Autodesk Inventor part; units mm, degrees
ref_plane "YZ Plane" through (0, 0, 0) normal (1, 0, 0) x (0, 1, 0)
ref_plane "XZ Plane" through (0, 0, 0) normal (0, 1, 0) x (-1, 0, 0)
ref_plane "XY Plane" through (0, 0, 0) normal (0, 0, 1) x (1, 0, 0)
sketch "草圖1" plane through (0, 0, 0) normal (0, 1, 0) x (-1, 0, 0)
  line L0 (4.2, 0) -> (4.2, -6)
  line L1 (4.2, -6) -> (0, -6)
  line L2 (0, -6) -> (1.2, -6)
  line L3 (1.2, -6) -> (1.2, -12)
  line L4 (1.2, -12) -> (0, -12)
  line L5 (-4.2, 0) -> (-4.2, -6)
  line L6 (-4.2, -6) -> (0, -6)
  line L7 (0, -6) -> (-1.2, -6)
  line L8 (-1.2, -6) -> (-1.2, -12)
  line L9 (-1.2, -12) -> (0, -12)
  line L10 (4.2, 0) -> (4.2, 6)
  line L11 (4.2, 6) -> (0, 6)
  line L12 (0, 6) -> (1.2, 6)
  line L13 (1.2, 6) -> (1.2, 12)
  line L14 (1.2, 12) -> (0, 12)
  line L15 (-4.2, 0) -> (-4.2, 6)
  line L16 (-4.2, 6) -> (0, 6)
  line L17 (0, 6) -> (-1.2, 6)
  line L18 (-1.2, 6) -> (-1.2, 12)
  line L19 (-1.2, 12) -> (0, 12)
  circle A0 centre (0, 0) radius 1.5
  dimension "d0" = 6
  dimension "d1" = 1.2
  dimension "d2" = 3
  dimension "d3" = 6
  dimension "d4" = 3
extrude "擠出1" add sketch "草圖1" along normal mid plane 3
properties part number "小零件1"
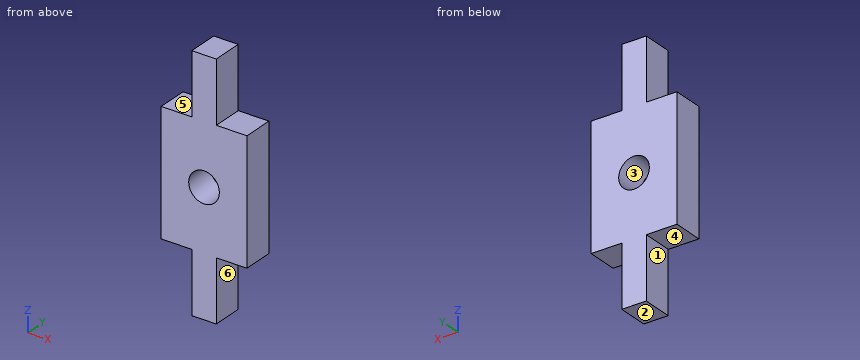
Source: CAD feature listing. Evaluate the final solid. Frame: model axes, mm. Face numbers are marked on the shaded views. A direction names the side the tool comes from. Give positions to 0.01 mm unless a question says otherwise; leave off trailing zeros. Write each loop counter-clockwise with the first axis right and the second up, starting at its lowest first coordinate (ties: lowest second). Pieces come first, ordered by that corner, then holes.
1. Material intervals for line 1 along Z through (x, y) = (0, 0.7); line 2 along Z through (x, y) = (2.75, -0.35); line 3 along X through (y, z) = (0.7, 1), sorted ascending.
2. First-contact query: pin 1 (1.5 mm diameter, centred on y = -0.5, z = 10.5, fed in from +X); pin 2 (0.9 mm diameter, centred on x = 3.5, y = 0.5, fed in from -Z); pin 3 (1.5 mm diameter, centred on y = 0.5, z = -9.5, fed in from -X). Flat tips, straight axial feed; report the tip coordinate or a pass-through.
3. Pull-direction query (X, two-part tool) for the marked faces 1, 2 and 3; classes: +X half, -X half, draft (parallel to the pull), parting line (faces both ways), or undercut.
4. Section query B-B (y = 0.15). Return the cut outline in (x, z).
5. Section query A-A (z = 0). Return the cut outline in (x, y), then the cut area to 3 significant figures.
6. Access query for the marked faces 4, 5 and 6. Directions: +Z, -Z, +X, -X, +Y, -Y. A direction counts if a zero-diameter tool reaches every point of the face in a straight line with its end or side. Return the directions, or none.
7. Section query D-D (x = -2). Return the cut outline in (y, z).
8. Section query C-C (x = 0). Return the cut outline in (y, z), then the cut area to 3 significant figures.
Output values:
1. line 1: z = -12 to -1.5, 1.5 to 12
1. line 2: z = -6 to 6
1. line 3: x = -4.2 to -1.12, 1.12 to 4.2
2. pin 1: stops at x = 1.2
2. pin 2: stops at z = -6
2. pin 3: stops at x = -1.2
3. face 1: -X half
3. face 2: draft
3. face 3: undercut
4. outline: (-4.2, -6) - (-1.2, -6) - (-1.2, -12) - (1.2, -12) - (1.2, -6) - (4.2, -6) - (4.2, 6) - (1.2, 6) - (1.2, 12) - (-1.2, 12) - (-1.2, 6) - (-4.2, 6) - close; hole circle Ø3 at (0, 0)
5. outline: (-4.2, -1.5) - (-1.5, -1.5) - (-1.5, 1.5) - (-4.2, 1.5) - close; (1.5, -1.5) - (4.2, -1.5) - (4.2, 1.5) - (1.5, 1.5) - close
5. area: 16.2 mm2
6. face 4: -Z, -X, +Y, -Y
6. face 5: +Z, -X, +Y, -Y
6. face 6: -Z, +X, +Y, -Y
7. outline: (-1.5, -6) - (1.5, -6) - (1.5, 6) - (-1.5, 6) - close
8. outline: (-1.5, -12) - (1.5, -12) - (1.5, -1.5) - (-1.5, -1.5) - close; (-1.5, 1.5) - (1.5, 1.5) - (1.5, 12) - (-1.5, 12) - close
8. area: 63.0 mm2
